Input: part model. Units: mm. Frame: model coordinates. A direction names the side the tool comes from. Coordinates: 2 decimals unless noted, no trailing zeros. Write each loop counter-clockwise with the first axis right and the second up, starting at its lowest first coordinate (ties: lowest second). Pieces come first, ordered by that corner, then holes.
from build123d import *

# Parameters (mm, degrees)
EXTRUDE_1_DEPTH     = 4
CUT_EXTRUDE_1_DEPTH = 1.5
SKETCH_2_R          = 4
EXTRUDE_2_DEPTH     = 20
CUT_EXTRUDE_2_DEPTH = 5
CHAMFER_2_SIZE      = 1


with BuildPart() as part:
    # Эскиз1 → Бобышка-Вытянуть1 (new body, symmetric)
    with BuildSketch(Plane.XY):
        Polygon((8.9, 0), (-8.9, 0), (-8.9, 4), (-4, 4), (-4, 5.5), (4, 5.5), (4, 4), (8.9, 4), align=None)
    extrude(amount=EXTRUDE_1_DEPTH, both=True)

    # Эскиз3 → Вырез-Вытянуть1 (cut)
    with BuildSketch(Plane(origin=(0, 5.5, 0), x_dir=(1, 0, 0), z_dir=(0, 1, 0))):
        with BuildLine():
            Line((-4, 0), (-4, 4))
            Line((-4, 4), (0, 4))
            ThreePointArc((0, 4), (-2.828427125, 2.828427125), (-4, 0))
        make_face()
        with BuildLine():
            Line((0, -4), (4, -4))
            Line((4, -4), (4, 0))
            ThreePointArc((4, 0), (2.828427125, -2.828427125), (0, -4))
        make_face()
    extrude(amount=-CUT_EXTRUDE_1_DEPTH, mode=Mode.SUBTRACT)

    # Эскиз2 → Бобышка-Вытянуть2 (add)
    with BuildSketch(Plane(origin=(0, 5.5, 0), x_dir=(1, 0, 0), z_dir=(0, 1, 0))):
        with Locations(Location((0, 0, 0), (0, 0, 270))):  # turned: the seam where the file's is
            Circle(SKETCH_2_R)
    extrude(amount=EXTRUDE_2_DEPTH)

    # Эскиз4 → Вырез-Вытянуть2 (cut, through all)
    with BuildSketch(Plane(origin=(0, 4, 0), x_dir=(1, 0, 0), z_dir=(0, 1, 0))):
        with BuildLine():
            Line((-7.950471684, 4), (-8.9, 4))
            Line((-8.9, 4), (-8.9, 0))
            ThreePointArc((-8.9, 0), (-8.659364815, 2.055578022), (-7.950471684, 4))
        make_face()
        with BuildLine():
            Line((7.950471684, -4), (8.9, -4))
            Line((8.9, -4), (8.9, 0))
            ThreePointArc((8.9, 0), (8.659364815, -2.055578022), (7.950471684, -4))
        make_face()
    extrude(amount=-CUT_EXTRUDE_2_DEPTH, mode=Mode.SUBTRACT)

    # Вырез-По траектории1: sweep along a path in Эскиз6
    with BuildLine(Plane.XZ) as sweep_1_path:
        Line((0, -8.9), (8.9, -8.9))
        Line((8.9, -8.9), (8.9, 0))
        ThreePointArc((8.9, 0), (6.293250353, 6.293250353), (0, 8.9))
        Line((0, 8.9), (-8.9, 8.9))
        Line((-8.9, 8.9), (-8.9, 0))
        ThreePointArc((-8.9, 0), (-6.293250353, -6.293250353), (0, -8.9))
    # Эскиз5 → Вырез-По траектории1 (sweep, cut)
    with BuildSketch(Plane.XY.offset(4)):
        Polygon((-8.9, 2.5), (-4.8, 0), (-8.9, 0), align=None)
    sweep(path=sweep_1_path.line, transition=Transition.RIGHT, mode=Mode.SUBTRACT)

    # Фаска2
    chamfer_2_edges = [part.edges().sort_by_distance(p)[0] for p in [
        (0, 25.5, -4),
    ]]
    chamfer(chamfer_2_edges, length=CHAMFER_2_SIZE)


solid = part.part
Item 1: Pin query (flat end, axial travel): pin 1 Ø0.8 at (y, z) = (4.5, 1.5) entering from -X; pin 2 Ø4 at (x, y) = (6.5, 12) entering from +Z; pin 3 Ø1 at (x, z) = (6, 2) entering from -Y; pin 4 Ø2 at (x, y) = (-3.5, 9) entering from -Z. Return the tip coordinate at first contact, or that it passes through.
Item 2: Section query A-A, the plane y = 1.75. Return loops of the section in (x, z).
Item 3: Section query B-B, the plane y = 18.5. Return loops of the section in (x, z).
Item 4: Access query for faces 1 (the face through (-4, 5, 2)), 2 (the face through (3, 5.5, -3)), 3 (the face through (-3, 5.5, 3)). Directions: +Z, -Z, +X, -X, +Y, -Y. A direction counts if a zero-diameter tool reaches every point of the face in a straight line with its end or side. Return the directions, or none.
Item 5: Material intervals for line 1 (X direction, y = 22.25, z = -2.25); line 2 (Z direction, x = -2.5, y = 16); line 3 (Y direction, x = 6, z = 3.25), sorted ascending.
The answers:
1. pin 1: stops at x = -4
1. pin 2: passes through
1. pin 3: stops at y = 0.62
1. pin 4: stops at z = -3.12
2. outline: (-7.67, 0) arc R7.67 ccw to (-6.54, -4) - (7.67, -4) - (7.67, 0) arc R7.67 ccw to (6.54, 4) - (-7.67, 4) - close
3. outline: circle Ø8 at (0, 0)
4. face 1: +Z, -Z, -X, +Y
4. face 2: -Z, +X, +Y
4. face 3: +Z, -X, +Y
5. line 1: x = -3.31 to 3.31
5. line 2: z = -3.12 to 3.12
5. line 3: y = 1.23 to 4
